The listing builds one solid part. Answer for the finished solid, in the listing's coordinates (mm). A direction names the side the tool comes from. Give positions to 0.01 mm unless a question says otherwise; leave off trailing zeros. Write each loop counter-clockwise with the first axis right and the second up, starting at its lowest first coordinate (ties: lowest second). Pieces come first, ordered by that corner, then holes.
Autodesk Inventor part; units mm, degrees
ref_plane "YZ Plane" through (0, 0, 0) normal (1, 0, 0) x (0, 1, 0)
ref_plane "XZ Plane" through (0, 0, 0) normal (0, 1, 0) x (-1, 0, 0)
ref_plane "XY Plane" through (0, 0, 0) normal (0, 0, 1) x (1, 0, 0)
sketch "Náčrt1" plane through (0, 0, 0) normal (0, 0, 1) x (1, 0, 0)
  line L0 (0, 95.014) -> (0, -94.5857)
  line L1 (-94.5, 0) -> (94.5, 0)
  circle A0 centre (0, 0) radius 63.5
  arc A1 (-53.5, 41.1582) -> (53.5, 41.1582) centre (0, 0) ccw
  line L2 (-18.2003, 65) -> (18.2003, 65)
  arc A2 (53.8673, 40.6764) -> (18.2003, 65) centre (0, 0) ccw
  arc A3 (-18.2003, 65) -> (-53.5, 41.1582) centre (0, 0) ccw
  point P0 (53.5, 41.1582)
  dimension "d0" = 127
  dimension "d1" = 135
  dimension "d2" = 107
  dimension "d8" = 65
extrude "Vysunutí1" add sketch "Náčrt1" along normal blind 3
sketch "Náčrt2" plane through (0, 0, 3) normal (0, 0, 1) x (1, 0, 0)
  circle A0 centre (0, 0) radius 63.5
  arc A1 (-18.2003, 65) -> (18.2003, 65) centre (0, 0) ccw
  line L0 (18.2003, 65) -> (-18.2003, 65)
  line L1 (-18.2003, 65) -> (18.2003, 65)
  line L2 (18.2003, 65) -> (-18.2003, 65)
  circle A2 centre (0, 0) radius 67.5
  circle A3 centre (0, 0) radius 63.5
  point P0 (53.5, 72.3723)
  point P1 (-53.5, 72.3723)
  dimension "d5" = 127
extrude "Vysunutí2" add sketch "Náčrt2" along normal blind 30 contours L0 A1
properties part number "Miska"
Item 1: A cutting plane is placed at D-D, the plane x = -27. Give the vertices of the cut face in (y, z), plus the area to 3 significant figures.
Conclusion:
outline: (-61.86, 0) - (61.86, 0) - (61.86, 33) - (57.47, 33) - (57.47, 3) - (-57.47, 3) - (-57.47, 33) - (-61.86, 33) - close
area: 635 mm2
Item 2: A cutting plane is placed at C-C, the plane x = -9.5. Give the vertices of the cut face in (y, z).
Conclusion:
outline: (-66.83, 0) - (65, 0) - (65, 33) - (62.79, 33) - (62.79, 3) - (-62.79, 3) - (-62.79, 33) - (-66.83, 33) - close
Item 3: Which of the six approach directions +Z, -Z, +X, -X, +Y, -Y give full straight-line access (tool end or side, diameter ignored) to faces 4 (the face through (-13.77, 61.99, 17.79)), 5 (the face through (0, 65, 16))?
Conclusion:
face 4: +Z
face 5: +Z, -Z, +X, -X, +Y
Item 4: A cutting plane is placed at A-A, the plane z = 30.5. Give the vertices of the cut face in (x, y).
Conclusion:
outline: (-18.2, 65) arc R67.5 ccw (long way) to (18.2, 65) - close; hole circle Ø127 at (0, 0)
Item 5: A cutting plane is placed at B-B, the plane y = 0. Give the vertices of the cut face in (x, z), plus the area to 3 significant figures.
Conclusion:
outline: (-67.5, 0) - (67.5, 0) - (67.5, 33) - (63.5, 33) - (63.5, 3) - (-63.5, 3) - (-63.5, 33) - (-67.5, 33) - close
area: 645 mm2
Item 6: Determine the mould class of faces 1 (the face through (-1, 1, 3)), 2 (the face through (37.528, 56.106, 1.479)), 3 (the face through (40, -50, 33)) for opening direction Y: pulls with the +Y half, pulls with the -Y half, needs draft (parallel to the pull), parting line crosses it, or undercut.
Conclusion:
face 1: undercut
face 2: pulls with the +Y half
face 3: needs draft
Item 7: Each of these flat-tipped pins is pushed along its axis until it touches: P1, Ø5, axis at x = 3.5, z = 16.5, coming from the -Y side; P2, Ø2, axis at x = 52.5, z = 16, coming from the +Y side; P3, Ø4, axis at x = -14, y = -25.5, coming from the +Z side; P4, Ø1, axis at x = -23.5, y = -46, coming from the -Z side. Where does it stop, or does it pass through?
Conclusion:
P1: stops at y = -67.49
P2: stops at y = 43.63
P3: stops at z = 3
P4: stops at z = 0
Item 8: Consider probe 1 along Y at (x, z) = (0, 24); probe 2 along Z at (x, y) = (9, 10.5); probe 3 along Y at (x, z) = (-14, 19). Determine where each line is inside the solid, lowest interval first.
Conclusion:
probe 1: y = -67.5 to -63.5, 63.5 to 65
probe 2: z = 0 to 3
probe 3: y = -66.03 to -61.94, 61.94 to 65
